Here's how the part is built. I have some questions about the finished solid (model axes, mm). Face numbers are marked on the shaded views. A direction names the side the tool comes from. Coordinates: 2 decimals unless noted, no trailing zeros. Write each loop counter-clockwise with the first axis right and the second up, starting at its lowest first coordinate (ties: lowest second). Pieces come first, ordered by that corner, then holes.
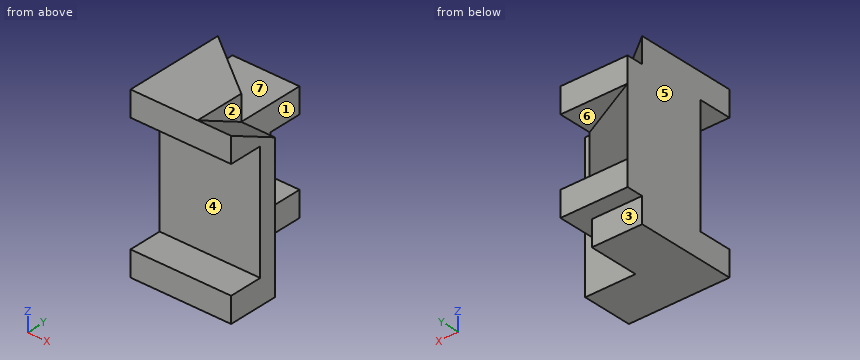
```python
from build123d import *

# Parameters (mm, degrees)
SALIENTE_EXTRUIR2_DEPTH = 6
CORTAR_EXTRUIR2_DEPTH   = 2
CROQUIS6_W              = 4
CROQUIS6_H              = 8
SALIENTE_EXTRUIR3_DEPTH = 4
CORTAR_EXTRUIR3_DEPTH   = 1.5
CROQUIS9_W              = 4
CROQUIS9_H              = 2
CORTAR_EXTRUIR4_DEPTH   = 5
CROQUIS10_W             = 1.5
CROQUIS10_H             = 4
SALIENTE_EXTRUIR4_DEPTH = 4
SALIENTE_EXTRUIR5_DEPTH = 4
CROQUIS13_W             = 3
CROQUIS13_H             = 3
SALIENTE_EXTRUIR6_DEPTH = 1.5


with BuildPart() as part:
    # Croquis2 → Saliente-Extruir2 (new body)
    with BuildSketch(Plane(origin=(0, 0, 0), x_dir=(0, 0, -1), z_dir=(1, 0, 0))):
        Polygon((0, 0), (0, -3), (1.5, -3), (1.5, -1), (8.5, -1), (8.5, -3), (10, -3), (10, 0), align=None)
    extrude(amount=SALIENTE_EXTRUIR2_DEPTH)

    # Croquis5 → Cortar-Extruir2 (cut)
    with BuildSketch(Plane(origin=(6, 0, 0), x_dir=(0, 0, -1), z_dir=(1, 0, 0))):
        Polygon((0, -3), (1.5, 0), (0, 0), align=None)
    extrude(amount=-CORTAR_EXTRUIR2_DEPTH, mode=Mode.SUBTRACT)

    # Croquis6 → Saliente-Extruir3 (add)
    with BuildSketch(Plane(origin=(0, 0, 0), x_dir=(1, 0, 0), z_dir=(0, 1, 0))):
        with Locations((2, 4)):
            Rectangle(CROQUIS6_W, CROQUIS6_H)
    extrude(amount=SALIENTE_EXTRUIR3_DEPTH)

    # Croquis7 → Cortar-Extruir3 (cut)
    with BuildSketch(Plane.XY):
        Polygon((0, 3), (4, 0), (4, 4), (0, 4), align=None)
    extrude(amount=-CORTAR_EXTRUIR3_DEPTH, mode=Mode.SUBTRACT)

    # Croquis9 → Cortar-Extruir4 (cut)
    with BuildSketch(Plane(origin=(4, 0, 0), x_dir=(0, 0, -1), z_dir=(1, 0, 0))):
        with Locations((5, 3)):
            Rectangle(CROQUIS9_W, CROQUIS9_H)
    extrude(amount=-CORTAR_EXTRUIR4_DEPTH, mode=Mode.SUBTRACT)

    # Croquis10 → Saliente-Extruir4 (add)
    with BuildSketch(Plane(origin=(4, 0, 0), x_dir=(0, 0, -1), z_dir=(1, 0, 0))):
        with Locations((7.75, 2)):
            Rectangle(CROQUIS10_W, CROQUIS10_H)
    extrude(amount=-SALIENTE_EXTRUIR4_DEPTH)

    # Croquis12 → Saliente-Extruir5 (add)
    with BuildSketch(Plane.XY.offset(-7)):
        Polygon((0, 4), (4, 2), (0, 2), align=None)
    extrude(amount=SALIENTE_EXTRUIR5_DEPTH)

    # Croquis13 → Saliente-Extruir6 (add)
    with BuildSketch(Plane(origin=(0, 0, -8.5), x_dir=(-1, 0, 0), z_dir=(0, 0, -1))):
        with Locations((-1.5, 1.5)):
            Rectangle(CROQUIS13_W, CROQUIS13_H)
    extrude(amount=SALIENTE_EXTRUIR6_DEPTH)


solid = part.part
```
1) Imagine slicing it at C-C on z = -3.5. Please give me the cut outline in (x, y), then the cut area to 3 significant figures.
Values follow:
outline: (0, -1) - (6, -1) - (6, 0) - (4, 0) - (4, 2) - (0, 4) - close
area: 18.0 mm2
2) I need wall thicknesses on probe 1 along Z at (x, y) = (2.55, -1.75); probe 2 along Z at (x, y) = (3.4, 3); probe 3 along X at (y, z) = (1.5, -2.5). Which ranges of each line are inside material? Lowest first, please.
Values follow:
probe 1: z = -10 to -8.5, -1.5 to 0
probe 2: z = -8.5 to -7, -3 to -1.5
probe 3: x = 0 to 4
3) We'd pull the mould along Z, two halves only. Please class the marked faces 5, 6 and 7: pulls with the +Z half, pulls with the -Z half, needs draft (parallel to the pull), parting line crosses it, or undercut.
Values follow:
face 5: needs draft
face 6: undercut
face 7: pulls with the +Z half
4) Imagine slicing it at D-D on y = 2.5. Please give me the cut outline in (x, z), then the cut area to 3 significant figures.
Values follow:
outline: (0, -10) - (3, -10) - (3, -8.5) - (4, -8.5) - (4, -7) - (3, -7) - (3, -3) - (4, -3) - (4, -1.5) - (0.67, -1.5) - (0.67, 0) - (0, 0) - close
area: 29.5 mm2
5) On a 3-axis mill with a long thin cutter (end or side, diameter ignored), from which of +Z, -Z, +X, -X, +Y, -Y can I reach the whole of each face in a straight line? I mean the marked faces 1, 2, 3 and 4. Say none if no direction works.
Values follow:
face 1: +Z, -Z, +X, +Y
face 2: +Z, +X, +Y
face 3: -Z, +X, -X, +Y
face 4: +X, -X, -Y
6) Imagine slicing it at A-A on x = 1. Please give me the cut outline in (y, z), then the cut area to 3 significant figures.
Values follow:
outline: (-3, -10) - (3, -10) - (3, -8.5) - (4, -8.5) - (4, -7) - (3.5, -7) - (3.5, -3) - (4, -3) - (4, -1.5) - (2.25, -1.5) - (2.25, 0) - (-3, 0) - (-3, -1.5) - (-1, -1.5) - (-1, -8.5) - (-3, -8.5) - close
area: 49.9 mm2
7) Will these pins go through, and if not, where does the flat tip stop? pin 1 (1.5 mm diameter, centred on x = 3, y = 3, fed in from +Z); pin 2 (1.5 mm diameter, centred on x = 5, z = -4, fed in from +Y); pin 3 (1.6 mm diameter, centred on x = 1.5, z = -9.5, fed in from +Y).
Values follow:
pin 1: stops at z = -1.5
pin 2: stops at y = 0
pin 3: stops at y = 3
8) Imagine slicing it at B-B on y = -2. Please give me the cut outline in (x, z), then the cut area to 3 significant figures.
Values follow:
outline: (0, -10) - (6, -10) - (6, -8.5) - (0, -8.5) - close; (0, -1.5) - (6, -1.5) - (6, -0.5) - (4, -0.5) - (4, 0) - (0, 0) - close
area: 17.0 mm2
